Read the model definition and answer for the solid it produces. Units are mm, in the model's axes. Face numbers are marked on the shaded views. A direction names the side the tool comes from. Give positions to 0.01 mm unless a question says otherwise; leave off trailing zeros. Order: outer loops, then holes, each group sorted by start corner. A loop starts at its lowest first (then second) coordinate and runs counter-clockwise, first axis right, second up. Notation, with made-up numbers: (-18, 34) - (18, 34) arc R28 ccw to (18, 59) - close; hole circle Ø7 at (60, 53.25). An arc over 180 degrees is marked (long way). Use a Markdown table: item, result. Add a question column.
1. Which of the six approach directions +Z, -Z, +X, -X, +Y, -Y give full straight-line access (tool end or side, diameter ignored) to the marked faces 1 and 2?
2. A cutting plane is placed at A-A on y = 0. Determine the outline of the cut face in (x, z).
3. A cutting plane is placed at C-C on x = -97. Determine the outline of the cut face in (y, z), and give its area (3 significant figures).
4. Consider L1, parallel to X at y = -31.5, z = 0; L2, parallel to Y at x = -119, z = 12; L3, parallel to X at y = -19.5, z = 44. Determine where each line is inside the solid, lowest interval first.
5. A cutting plane is placed at D-D on x = -22.5. Determine the outline of the cut face in (y, z), and give its area (3 significant figures).
6. Flat-ended cylindrical pins translate along their axes: P1, Ø5, axis at x = -74, y = 7, coming from the +Z side; P2, Ø6, axis at y = -45.5, z = -43, coming from the +X side; P3, Ø8, axis at y = 5.5, z = -54, coming from the -X side. Find the tip coordinate at first contact, or state that the pin passes through.
```python
from build123d import *

# Parameters (mm, degrees)
F2_R = 3


with BuildPart() as f1:
    # F0 (on Front) → F1 (revolve)
    with BuildSketch(Plane.XZ):
        Polygon((-160, 15), (-160, 0), (0, 0), (0, 42.460439), (-24.814942, 80), (-24.814942, 42.460439), (-30.361943, 34.139935), (-135, 34.139935), (-135, 15), align=None)
    revolve(axis=Axis((-80, 0, 0), (-1, 0, 0)))

    # F2
    f2_edges = [f1.edges().sort_by_distance(p)[0] for p in [
        (-135, 0, -34.139935),
        (-135, 0, -15),
    ]]
    fillet(f2_edges, radius=F2_R)


solid = f1.part
```
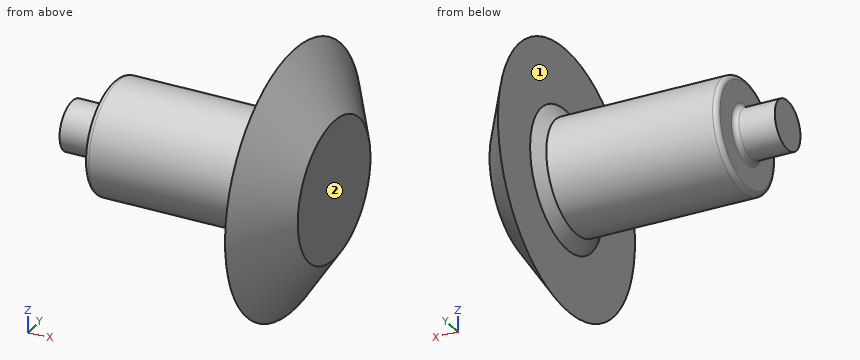
Output values:
| question | item | result |
|---|---|---|
| 1 | face 1 | -X |
| 1 | face 2 | +Z, -Z, +X, +Y, -Y |
| 2 | outline | (-160, -15) - (-138, -15) arc R3 cw to (-135, -18) - (-135, -31.14) arc R3 ccw to (-132, -34.14) - (-30.36, -34.14) - (-24.81, -42.46) - (-24.81, -80) - (0, -42.46) - (0, 42.46) - (-24.81, 80) - (-24.81, 42.46) - (-30.36, 34.14) - (-132, 34.14) arc R3 ccw to (-135, 31.14) - (-135, 18) arc R3 cw to (-138, 15) - (-160, 15) - close |
| 3 | outline | circle Ø68.28 at (0, 0) |
| 3 | area | 3,660 mm² |
| 4 | L1 | -134.98 to 0 |
| 4 | L2 | -31.96 to 31.96 |
| 4 | L3 | -24.81 to -3.75 |
| 5 | outline | circle Ø153 at (0, 0) |
| 5 | area | 18,400 mm² |
| 6 | P1 | z = 33.84 |
| 6 | P2 | x = -11.33 |
| 6 | P3 | x = -24.81 |
